```python
from build123d import *

# Parameters (mm, degrees)
F1_DEPTH = 25.4
F2_R     = 3.419127
F3_DEPTH = 31.496
F5_DEPTH = 36.322


with BuildPart() as f1:
    # F0 (on Top) → F1 (new body)
    with BuildSketch(Plane.XY):
        with BuildLine():
            ThreePointArc((-22.843207, -56.337804), (0, -79.181011), (22.843207, -56.337804))
            Line((22.843207, -56.337804), (7.287237, -56.337804))
            ThreePointArc((7.287237, -56.337804), (0, -63.625041), (-7.287237, -56.337804))
            Line((-7.287237, -56.337804), (-22.843207, -56.337804))
        make_face()
        with BuildLine():
            Line((7.287237, -56.337804), (22.843207, -56.337804))
            Line((22.843207, -56.337804), (22.843207, 56.337804))
            Line((22.843207, 56.337804), (7.301988, 56.337804))
            ThreePointArc((7.301988, 56.337804), (0, 49.035816), (-7.301988, 56.337804))
            Line((-7.301988, 56.337804), (-22.843207, 56.337804))
            Line((-22.843207, 56.337804), (-22.843207, -56.337804))
            Line((-22.843207, -56.337804), (-7.287237, -56.337804))
            ThreePointArc((-7.287237, -56.337804), (0, -49.050566), (7.287237, -56.337804))
        make_face()
        with BuildLine():
            Line((7.301988, 56.337804), (22.843207, 56.337804))
            ThreePointArc((22.843207, 56.337804), (0, 79.181011), (-22.843207, 56.337804))
            Line((-22.843207, 56.337804), (-7.301988, 56.337804))
            ThreePointArc((-7.301988, 56.337804), (0, 63.639791), (7.301988, 56.337804))
        make_face()
    extrude(amount=F1_DEPTH)

    # F2 (on Front) → F3 (join, symmetric)
    with BuildSketch(Plane.XZ):
        with BuildLine():
            Line((-9.637341, 25.398405), (9.637341, 25.398405))
            Line((9.637341, 25.398405), (9.637341, 43.869978))
            ThreePointArc((9.637341, 43.869978), (0, 53.507319), (-9.637341, 43.869978))
            Line((-9.637341, 43.869978), (-9.637341, 25.398405))
        make_face()
        with Locations((0, 43.869978)):
            Circle(F2_R, mode=Mode.SUBTRACT)
    extrude(amount=F3_DEPTH, both=True)

    # F4 (on Right) → F5 (cut, symmetric)
    with BuildSketch(Plane.YZ):
        with BuildLine():
            Line((11.288291, 41.059084), (11.645118, 41.059084))
            Line((11.645118, 41.059084), (11.645118, 65.955549))
            Line((11.645118, 65.955549), (-11.645118, 65.955549))
            Line((-11.645118, 65.955549), (-11.645118, 41.059084))
            Line((-11.645118, 41.059084), (-11.288291, 41.059084))
            ThreePointArc((-11.288291, 41.059084), (0, 29.770793), (11.288291, 41.059084))
        make_face()
    extrude(amount=F5_DEPTH, both=True, mode=Mode.SUBTRACT)


solid = f1.part
```
Could you check a few things on this model? Use its own coordinates, in mm. A direction names the side the tool comes from. Round coordinates to 2 decimals unless told otherwise and drop trailing zeros. Loops run counter-clockwise (first coordinate to the right, second up) from the corner with the lowest first, then second, coordinate; pieces in that order, holes last.
Q1. I want a section at D-D (y = 0). Write out the boundary of the cut face in (x, z).
Q2. Please list where these lines run through material, in increasing order: L1, parallel to Y at x = 0, z = 11.5; L2, parallel to Z at x = 0, y = -17; L3, parallel to Y at x = -5.5, z = 47.5.
Q3. Thinking about a two-plate mould opening in X: for faces 5 (the cylindrical face through (0.502, 79.175, 12.522)), 6 (the flat face through (0, -31.496, 40)), 7 (the cylindrical face through (-0.74, -21.24, 40.53)), which applies, pulls with the +X half, pulls with the -X half, needs draft (parallel to the pull), parting line crosses it, or undercut?
Q4. I want a section at C-C (z = 34). Write out the boundary of the cut face in (x, y).
Q5. On a 3-axis mill with a long thin cutter (end or side, diameter ignored), from which of +Z, -Z, +X, -X, +Y, -Y can I reach the whole of each face in a straight line? I mean faces 1 (the flat face through (9.637, 0, 28)), 2 (the flat face through (0, 11.645, 49)), 3 (the flat face through (0, 31.496, 40)), 4 (the flat face through (-9.637, 0, 29)). Say none if no direction works.
Q6. I want a section at A-A (x = 0). Write out the boundary of the cut face in (y, z), and give its area (3 significant figures).
Q7. For P1, Ø3.5, axis at x = -4, z = 46.5, coming from the +Y side; P2, Ø15.5, axis at x = -3, z = 36.5, coming from the -Y side; P3, Ø1.5, axis at x = 5.5, z = 22.5, coming from the -Y side, each with a flat end and sliding along its axis, tell me the tip position at first contact or that it passes through.
Q8. I want a section at B-B (z = 9). Write out the boundary of the cut face in (x, y), and give its area (3 significant figures).
Answer below:
1. outline: (-22.84, 0) - (22.84, 0) - (22.84, 25.4) - (9.64, 25.4) - (9.64, 29.77) - (-9.64, 29.77) - (-9.64, 25.4) - (-22.84, 25.4) - close
2. L1: y = -79.18 to -63.63, -49.05 to 49.04, 63.64 to 79.18
2. L2: z = 0 to 40.45, 47.29 to 53.51
2. L3: y = -31.5 to -11.65, 11.65 to 31.5
3. face 5: parting line crosses it
3. face 6: needs draft
3. face 7: undercut
4. outline: (-9.64, -31.5) - (9.64, -31.5) - (9.64, -8.81) - (-9.64, -8.81) - close; (-9.64, 8.81) - (9.64, 8.81) - (9.64, 31.5) - (-9.64, 31.5) - close
5. face 1: +Z, +X, +Y, -Y
5. face 2: +Z, +X, -X
5. face 3: +Z, +X, -X, +Y
5. face 4: +Z, -X, +Y, -Y
6. outline: (-79.18, 0) - (-63.63, 0) - (-63.63, 25.4) - (-79.18, 25.4) - close; (-49.05, 0) - (49.04, 0) - (49.04, 25.4) - (31.5, 25.4) - (31.5, 40.45) - (11.27, 40.45) arc R11.29 cw to (-11.27, 40.45) - (-31.5, 40.45) - (-31.5, 25.4) - (-49.05, 25.4) - close; (-31.5, 47.29) - (-11.65, 47.29) - (-11.65, 53.51) - (-31.5, 53.51) - close; (11.65, 47.29) - (31.5, 47.29) - (31.5, 53.51) - (11.65, 53.51) - close; (63.64, 0) - (79.18, 0) - (79.18, 25.4) - (63.64, 25.4) - close
6. area: 4,290 mm2
7. P1: stops at y = 31.5
7. P2: stops at y = -31.5
7. P3: stops at y = -78.68
8. outline: (-22.84, -56.34) arc R22.84 ccw to (22.84, -56.34) - (22.84, 56.34) arc R22.84 ccw to (-22.84, 56.34) - close; hole (-7.3, 56.34) arc R7.3 ccw to (7.3, 56.34) arc R7.3 ccw to start; hole circle Ø14.57 at (0, -56.34)
8. area: 6,450 mm2
